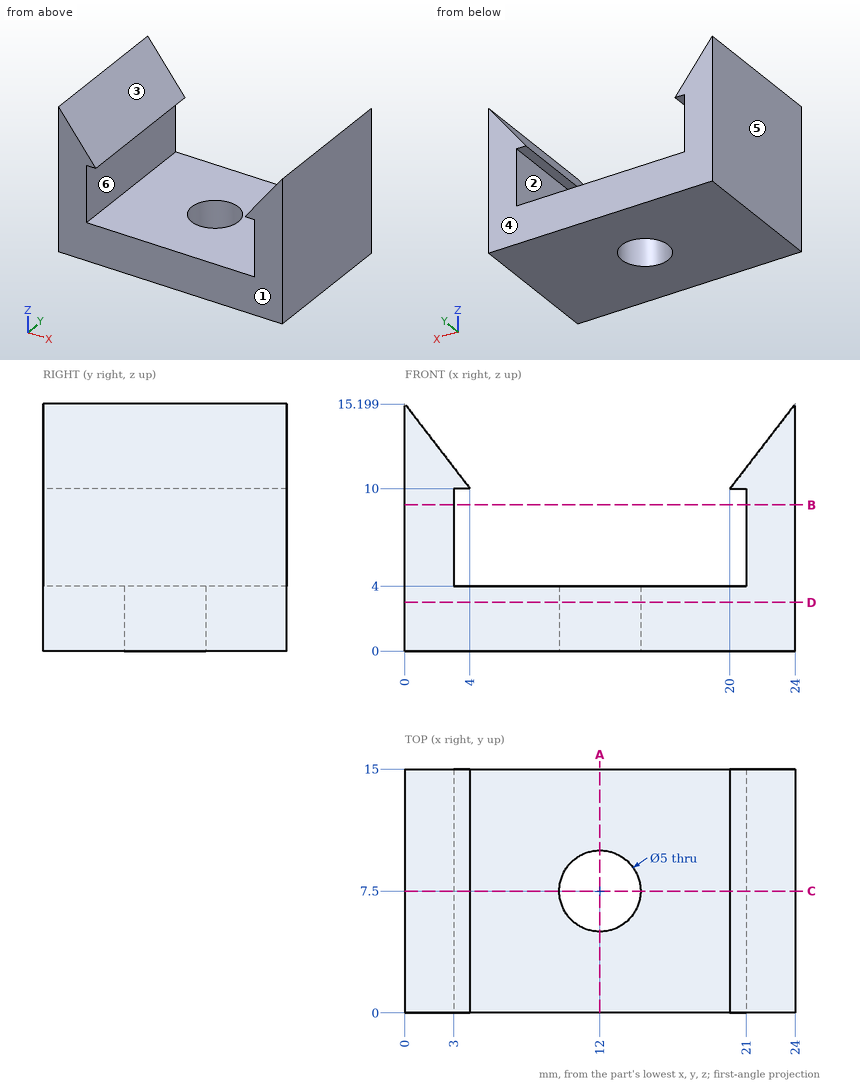
Print and shaded views of the part. All mm, measured from the part's lowest x, y and z. A direction names the side the tool comes from. Give positions to 0.01 mm unless a question says otherwise; leave off trailing zeros. Write each loop counter-clockwise with the first axis right and the second up, starting at its lowest first coordinate (ties: lowest second). Pieces come first, ordered by that corner, then holes. Notation, with made-up numbers: (89.5, -12.75) - (93.5, -12.75) arc R16 cw to (93.5, 6.25) - close; hole circle Ø9 at (-23.5, -27.5). An arc over 180 degrees is marked (long way). One line per question, with ' | ' between items. Start each with the question number.
(1) Pin check, flat tips, straight feed: P1, Ø5, axis at x = 4.5, y = 6, coming from the +Z side; P2, Ø4, axis at x = 9.5, y = 11, coming from the +Z side. Stop position of each tip, or through.
(2) Slice it at D-D on z = 3. Write the cut outline in (x, y), plus the area to 3 significant figures.
(3) Two-plate mould, pull along X, no slides. Class the marked faces 4, 5 and 6: +X half, -X half, draft (parallel to the pull), parting line (faces both ways), or undercut.
(4) Slice it at C-C on y = 7.5. Write the cut outline in (x, z).
(5) Slice it at A-A on x = 12. Write the cut outline in (y, z).
(6) Slice it at B-B on z = 9. Write the cut outline in (x, y).
(7) 3-axis set-ups, long thin cutter, end or side, ignore diameter. For the marked faces 1, 2 and 3: which of +Z, -Z, +X, -X, +Y, -Y reach the whole face in a straight line?
(8) Wall check: line 1 along Y through (x, z) = (12, 1.9); line 2 along X through (y, z) = (8.75, 4.5); line 3 along Z through (x, y) = (6.25, 11). Give the ranges that are in metal, low to high. Write a range as from..to.
Results below:
1) P1: z = 12.6 | P2: z = 4
2) outline: (0, 0) - (24, 0) - (24, 15) - (0, 15) - close; hole circle Ø5 at (12, 7.5) | area: 340 mm^2
3) face 4: draft | face 5: -X half | face 6: undercut
4) outline: (0, 0) - (9.5, 0) - (9.5, 4) - (3, 4) - (3, 10) - (4, 10) - (0, 15.2) - close; (14.5, 0) - (24, 0) - (24, 15.2) - (20, 10) - (21, 10) - (21, 4) - (14.5, 4) - close
5) outline: (0, 0) - (5, 0) - (5, 4) - (0, 4) - close; (10, 0) - (15, 0) - (15, 4) - (10, 4) - close
6) outline: (0, 0) - (3, 0) - (3, 15) - (0, 15) - close; (21, 0) - (24, 0) - (24, 15) - (21, 15) - close
7) face 1: +Z, -Z, +X, -X, -Y | face 2: +Y, -Y | face 3: +Z, +Y, -Y
8) line 1: 0..5, 10..15 | line 2: 0..3, 21..24 | line 3: 0..4
